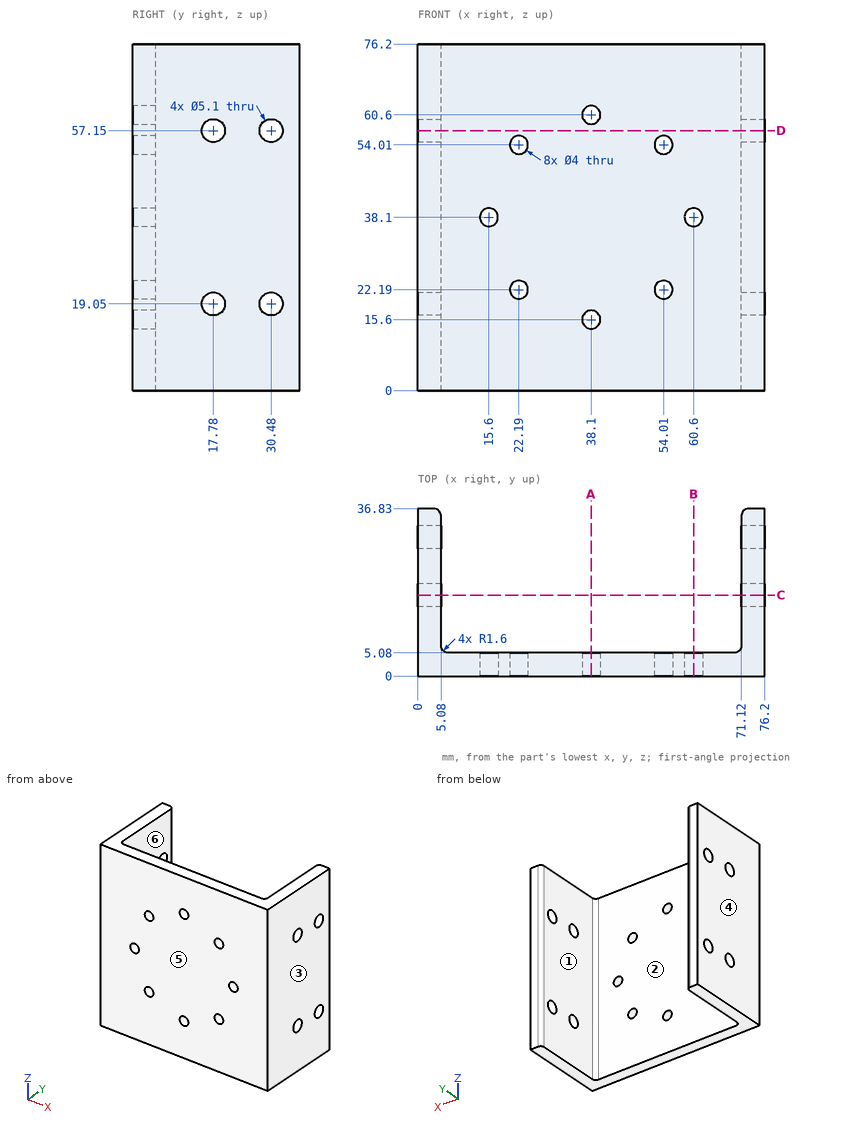
Could you check a few things on this drawing? It's one solid part, dimensions in mm from its lowest x, y, z. A direction names the side the tool comes from. Coordinates: 2 decimals unless noted, no trailing zeros. Loops run counter-clockwise (first coordinate to the right, second up) from the corner with the lowest first, then second, coordinate; pieces in that order, holes last. Notation, with made-up numbers: (41, 16) - (77, 16) arc R24 ccw to (77, 31) - close; hole circle Ø7 at (-26, 17.25). An arc over 180 degrees is marked (long way). Answer as a JSON object with one key per item and string values. Group by question number.
Item 1: On a 3-axis mill with a long thin cutter (end or side, diameter ignored), from which of +Z, -Z, +X, -X, +Y, -Y can I reach the whole of each face in a straight line? I mean the marked faces 5 and 6. Say none if no direction works.
Item 2: If we section it at B-B (x = 60.6): List the corners of the cut face in (y, z) for me.
Item 3: For pin 1 (6 mm diameter, centred on y = 17.78, z = 19.05, fed in from -X); pin 2 (3 mm diameter, centred on y = 30.48, z = 19.05, fed in from +X); pin 3 (6.5 mm diameter, centred on x = 38.1, z = 60.6, fed in from +Y), each with a flat end and sliding along its axis, tell me the tip position at first contact or that it passes through.
Item 4: If we section it at D-D (z = 57.15): List the corners of the cut face in (x, y) for me.
Item 5: If we mould it in two halves opening along X, with no side actions, what happens to the marked faces 1, 2, 3 and 4? For each: released by +X, released by -X, zero draft, split by the parting line, or undercut.
Item 6: If I drill on L1, parallel to Y at x = 2.9, z = 57.15; L2, parallel to X at y = 13.5, z = 71.5; L3, parallel to Y at x = 3, z = 58.5, over which ranges is the centre line in solid material (lowest first)? Write a range as from..to.
Item 7: If we section it at C-C (y = 17.78): List the corners of the cut face in (x, z) for me.
Item 8: If we section it at A-A (x = 38.1): List the corners of the cut face in (y, z) for me, plus the area to 3 significant figures.
Returned:
{
 "1": {"face 5": "+Z, -Z, +X, -X, -Y", "face 6": "+Z, -Z, +Y"},
 "2": {"outline": "(0, 0) - (5.08, 0) - (5.08, 36.1) - (0, 36.1) - close; (0, 40.1) - (5.08, 40.1) - (5.08, 76.2) - (0, 76.2) - close"},
 "3": {"pin 1": "stops at x = 0", "pin 2": "passes through", "pin 3": "stops at y = 5.08"},
 "4": {"outline": "(0, 0) - (76.2, 0) - (76.2, 15.23) - (71.12, 15.23) - (71.12, 6.68) arc R1.6 cw to (69.52, 5.08) - (6.68, 5.08) arc R1.6 cw to (5.08, 6.68) - (5.08, 15.23) - (0, 15.23) - close; (0, 20.33) - (5.08, 20.33) - (5.08, 27.93) - (0, 27.93) - close; (0, 33.03) - (5.08, 33.03) - (5.08, 35.23) arc R1.6 ccw to (3.48, 36.83) - (0, 36.83) - close; (71.12, 20.33) - (76.2, 20.33) - (76.2, 27.93) - (71.12, 27.93) - close; (71.12, 33.03) - (76.2, 33.03) - (76.2, 36.83) - (72.72, 36.83) arc R1.6 ccw to (71.12, 35.23) - close"},
 "5": {"face 1": "undercut", "face 2": "undercut", "face 3": "released by +X", "face 4": "released by -X"},
 "6": {"L1": "y = 0..15.23, 20.33..27.93, 33.03..36.83", "L2": "x = 0..5.08, 71.12..76.2", "L3": "y = 0..15.62, 19.94..28.32, 32.64..36.83"},
 "7": {"outline": "(0, 0) - (5.08, 0) - (5.08, 16.5) - (0, 16.5) - close; (0, 21.6) - (5.08, 21.6) - (5.08, 54.6) - (0, 54.6) - close; (0, 59.7) - (5.08, 59.7) - (5.08, 76.2) - (0, 76.2) - close; (71.12, 0) - (76.2, 0) - (76.2, 16.5) - (71.12, 16.5) - close; (71.12, 21.6) - (76.2, 21.6) - (76.2, 54.6) - (71.12, 54.6) - close; (71.12, 59.7) - (76.2, 59.7) - (76.2, 76.2) - (71.12, 76.2) - close"},
 "8": {"outline": "(0, 0) - (5.08, 0) - (5.08, 13.6) - (0, 13.6) - close; (0, 17.6) - (5.08, 17.6) - (5.08, 58.6) - (0, 58.6) - close; (0, 62.6) - (5.08, 62.6) - (5.08, 76.2) - (0, 76.2) - close", "area": "346 mm²"}
}
